from build123d import *

# Parameters (mm, degrees)
SKETCH2_R          = 3.175
CUT_EXTRUDE1_DEPTH = 96.882897328


with BuildPart() as part:
    # Sketch1 → Revolve2 (revolve)
    with BuildSketch(Plane.XY, mode=Mode.PRIVATE) as revolve2_sk:
        Polygon((19.05, 0), (50.8, 0), (50.8, 12.7), (25.4, 12.7), (25.4, 50.8), (50.8, 50.8), (50.8, 63.5), (19.05, 63.5), (19.05, 57.15), (6.35, 57.15), (6.35, 6.35), (19.05, 6.35), align=None)
    revolve(revolve2_sk.sketch.rotate(Axis((0, 0, 0), (0, 1, 0)), 90), axis=Axis((0, 0, 0), (0, 1, 0)))

    # Sketch2 → Cut-Extrude1 (cut, through all)
    with BuildSketch(Plane(origin=(0, 63.5, 0), x_dir=(1, 0, 0), z_dir=(0, 1, 0))):
        with Locations(Location((41.275, 0, 0), (0, 0, 270))):
            Circle(SKETCH2_R)
        with Locations(Location((29.185832393, -29.185832393, 0), (0, 0, 270))):
            Circle(SKETCH2_R)
        with Locations(Location((0, -41.275, 0), (0, 0, 270))):
            Circle(SKETCH2_R)
        with Locations(Location((-29.185832393, -29.185832393, 0), (0, 0, 270))):
            Circle(SKETCH2_R)
        with Locations(Location((-41.275, 0, 0), (0, 0, 270))):
            Circle(SKETCH2_R)
        with Locations(Location((-29.185832393, 29.185832393, 0), (0, 0, 270))):
            Circle(SKETCH2_R)
        with Locations(Location((0, 41.275, 0), (0, 0, 270))):
            Circle(SKETCH2_R)
        with Locations(Location((29.185832393, 29.185832393, 0), (0, 0, 270))):
            Circle(SKETCH2_R)
    extrude(amount=-CUT_EXTRUDE1_DEPTH, mode=Mode.SUBTRACT)


solid = part.part
Part model, mm, in its own coordinate system. A direction names the side the tool comes from. Coordinates: 2 decimals unless noted, no trailing zeros. Loops run counter-clockwise (first coordinate to the right, second up) from the corner with the lowest first, then second, coordinate; pieces in that order, holes last. Notation, with made-up numbers: (-28.75, 77.25) - (-19.75, 77.25) arc R28 cw to (-19.75, 95.25) - close; hole circle Ø9 at (43, 83). An arc over 180 degrees is marked (long way). Write each question's results on one line, items separated by ' | '. Start each with the question number.
Q1. Drop flat-ended pins along their axis: pin 1 Ø12 at (x, y) = (-2.5, 36) entering from -Z; pin 2 Ø5 at (y, z) = (10, 39) entering from -X; pin 3 Ø11.5 at (x, z) = (-9, -3) entering from +Y. Give the stop position or say it passes through.
Q2. Slice it at D-D on y = 34. Give the cut face in (x, z).
Q3. Slice it at B-B on z = -42. Give the cut face in (x, y), and give its area (3 significant figures).
Q4. Slice it at A-A on x = 0. Give the number of separate pieces and of enclosed holes in the cut face, and give its area (3 significant figures).
Q5. Two-plate mould, pull along X, no slides. Class faces 5 (the cylindrical face through (43.95, 6.44, 1.71)), 6 (the cylindrical face through (0.1, 6.4, 38.1)), 7 (the flat face through (-1, 0, 22)), 8 (the cylindrical face through (30.911, 6.439, 40.313)): +X half, -X half, draft (parallel to the pull), parting line (faces both ways), or undercut.
Q6. Probe line 1 along Y through (x, z) = (-42, 8); line 2 along Z through (x, y) = (31, 4.5); line 3 along Y through (x, z) = (-2, -11). List the from-to ranges inside material, lowest first.
Q7. Which spindle directions (+Z, -Z, +X, -X, +Y, -Y) get a long thin tool onto all of the face, cutting with end or side? Do faces 1 (the cylindrical face through (26.37, 57.24, 30.65)), 2 (the flat face through (-5, 57.15, 5)), 3 (the flat face through (-23.3, 50.8, 10.6)), 4 (the flat face through (-5, 6.35, -5)). Say none if no direction does.
Answer:
1) pin 1: stops at z = -25.4 | pin 2: stops at x = -35.33 | pin 3: stops at y = 57.15
2) outline: circle Ø50.8 at (0, 0); hole circle Ø12.7 at (0, 0)
3) outline: (-28.58, 0) - (-3.09, 0) - (-3.09, 12.7) - (-28.58, 12.7) - close; (-28.58, 50.8) - (-3.09, 50.8) - (-3.09, 63.5) - (-28.58, 63.5) - close; (3.09, 0) - (28.58, 0) - (28.58, 12.7) - (3.09, 12.7) - close; (3.09, 50.8) - (28.58, 50.8) - (28.58, 63.5) - (3.09, 63.5) - close | area: 1,290 mm2
4) separate pieces: 6 | enclosed holes: 0 | area: 3,060 mm2
5) face 5: undercut | face 6: undercut | face 7: draft | face 8: parting line
6) line 1: y = 0 to 12.7, 50.8 to 63.5 | line 2: z = -40.24 to -31.79, -26.58 to 26.58, 31.79 to 40.24 | line 3: y = 6.35 to 57.15
7) face 1: +Y, -Y | face 2: +Y | face 3: none | face 4: -Y
